```python
from build123d import *

# Parameters (mm, degrees)
SKETCH2_W           = 25
SKETCH2_H           = 42
BOSS_EXTRUDE1_DEPTH = 36
SKETCH4_W           = 23
SKETCH4_H           = 34
CUT_EXTRUDE2_DEPTH  = 61.704200843
FILLET2_R           = 2
SKETCH5_W           = 2.5
SKETCH5_H           = 10
CUT_EXTRUDE3_DEPTH  = 36
FILLET3_R           = 1
FILLET4_R           = 2
SKETCH7_W           = 6.678436395
SKETCH7_H           = 24
BOSS_EXTRUDE2_DEPTH = 2
FILLET5_R           = 2
SKETCH8_W           = 6.678436395
SKETCH8_H           = 2
BOSS_EXTRUDE5_DEPTH = 22
FILLET6_R           = 2
FILLET7_R           = 2
FILLET8_R           = 2
FILLET9_R           = 1
SKETCH10_R          = 2
SKETCH10_R_2        = 4
SKETCH10_R_3        = 1.5
CUT_EXTRUDE5_DEPTH  = 22
SKETCH11_R          = 2
CUT_EXTRUDE6_DEPTH  = 22
SKETCH14_R          = 1.480718613
SKETCH14_R_2        = 1.5
CUT_EXTRUDE8_DEPTH  = 1


with BuildPart() as part:
    # Sketch2 → Boss-Extrude1 (new body)
    with BuildSketch(Plane(origin=(0, 0, 0), x_dir=(1, 0, 0), z_dir=(0, 1, 0))):
        with Locations((12.5, 0)):
            Rectangle(SKETCH2_W, SKETCH2_H)
    extrude(amount=BOSS_EXTRUDE1_DEPTH)

    # Sketch4 → Cut-Extrude2 (cut, through all)
    with BuildSketch(Plane.XY.offset(21)):
        with Locations((13.5, 19)):
            Rectangle(SKETCH4_W, SKETCH4_H)
    extrude(amount=-CUT_EXTRUDE2_DEPTH, mode=Mode.SUBTRACT)

    # Fillet2
    fillet2_edges = [part.edges().sort_by_distance(p)[0] for p in [
        (25, 1, 21),
        (25, 1, -21),
    ]]
    fillet(fillet2_edges, radius=FILLET2_R)

    # Sketch5 → Cut-Extrude3 (cut)
    with BuildSketch(Plane(origin=(2, 0, 0), x_dir=(0, 0, -1), z_dir=(1, 0, 0))):
        with Locations((-19.75, 31)):
            Rectangle(SKETCH5_W, SKETCH5_H)
        with Locations((19.75, 31)):
            Rectangle(SKETCH5_W, SKETCH5_H)
    extrude(amount=-CUT_EXTRUDE3_DEPTH, mode=Mode.SUBTRACT)

    # Fillet3
    fillet3_edges = [part.edges().sort_by_distance(p)[0] for p in [
        (1, 26, 18.5),
        (1, 26, -18.5),
    ]]
    fillet(fillet3_edges, radius=FILLET3_R)

    # Fillet4
    fillet4_edges = [part.edges().sort_by_distance(p)[0] for p in [
        (1, 36, 18.5),
        (1, 36, -18.5),
    ]]
    fillet(fillet4_edges, radius=FILLET4_R)

    # Sketch7 → Boss-Extrude2 (add)
    with BuildSketch(Plane(origin=(2, 0, 0), x_dir=(0, 0, -1), z_dir=(1, 0, 0))):
        with Locations((-24.339218198, 19)):
            Rectangle(SKETCH7_W, SKETCH7_H)
        with Locations((24.339218198, 19)):
            Rectangle(SKETCH7_W, SKETCH7_H)
    extrude(amount=-BOSS_EXTRUDE2_DEPTH)

    # Fillet5
    fillet5_edges = [part.edges().sort_by_distance(p)[0] for p in [
        (1, 7, 27.678436395),
        (1, 7, -27.678436395),
    ]]
    fillet(fillet5_edges, radius=FILLET5_R)

    # Sketch8 → Boss-Extrude5 (add)
    with BuildSketch(Plane(origin=(2, 0, 0), x_dir=(0, 0, -1), z_dir=(1, 0, 0))):
        with Locations((-24.339218198, 30)):
            Rectangle(SKETCH8_W, SKETCH8_H)
        with Locations((24.339218198, 30)):
            Rectangle(SKETCH8_W, SKETCH8_H)
    extrude(amount=BOSS_EXTRUDE5_DEPTH)

    # Fillet6
    fillet6_edges = [part.edges().sort_by_distance(p)[0] for p in [
        (24, 30, 27.678436395),
        (24, 30, 21),
        (24, 30, -21),
        (24, 30, -27.678436395),
    ]]
    fillet(fillet6_edges, radius=FILLET6_R)

    # Fillet7
    fillet7_edges = [part.edges().sort_by_distance(p)[0] for p in [
        (0, 31, 24.339218197),
        (0, 31, -24.339218197),
    ]]
    fillet(fillet7_edges, radius=FILLET7_R)

    # Fillet8
    fillet8_edges = [part.edges().sort_by_distance(p)[0] for p in [
        (0, 0, 0),
    ]]
    fillet(fillet8_edges, radius=FILLET8_R)

    # Fillet9
    fillet9_edges = [part.edges().sort_by_distance(p)[0] for p in [
        (1, 26, 21),
        (1, 26, -21),
    ]]
    fillet(fillet9_edges, radius=FILLET9_R)

    # Sketch10 → Cut-Extrude5 (cut)
    with BuildSketch(Plane(origin=(2, 0, 0), x_dir=(0, 0, -1), z_dir=(1, 0, 0))):
        with Locations(Location((-22.678436395, 13, 0), (0, 0, 90))):
            Circle(SKETCH10_R)
        with Locations(Location((-22.678436395, 23, 0), (0, 0, 90))):
            Circle(SKETCH10_R)
        with Locations((22.678436395, 13)):
            Circle(SKETCH10_R)
        with Locations((22.678436395, 23)):
            Circle(SKETCH10_R)
        with Locations(Location((-11, 25, 0), (0, 0, 90))):
            Circle(SKETCH10_R_2)
        with Locations(Location((-11, 31.5, 0), (0, 0, 90))):
            Circle(SKETCH10_R_3)
        with Locations(Location((-11, 18.5, 0), (0, 0, 90))):
            Circle(SKETCH10_R_3)
        with Locations(Location((-17.5, 25, 0), (0, 0, 90))):
            Circle(SKETCH10_R_3)
        with Locations(Location((-4.5, 25, 0), (0, 0, 90))):
            Circle(SKETCH10_R_3)
        with Locations((11, 18.5)):
            Circle(SKETCH10_R_3)
        with Locations((4.5, 25)):
            Circle(SKETCH10_R_3)
        with Locations((17.5, 25)):
            Circle(SKETCH10_R_3)
        with Locations((11, 31.5)):
            Circle(SKETCH10_R_3)
        with Locations((11, 25)):
            Circle(SKETCH10_R_2)
        with Locations(Location((0, 15, 0), (0, 0, 90))):
            Circle(SKETCH10_R_2)
        with Locations(Location((6.5, 15, 0), (0, 0, 90))):
            Circle(SKETCH10_R_3)
        with Locations(Location((0, 8.5, 0), (0, 0, 90))):
            Circle(SKETCH10_R_3)
        with Locations(Location((0, 21.5, 0), (0, 0, 90))):
            Circle(SKETCH10_R_3)
        with Locations((-6.5, 15)):
            Circle(SKETCH10_R_3)
    extrude(amount=-CUT_EXTRUDE5_DEPTH, mode=Mode.SUBTRACT)

    # Sketch11 → Cut-Extrude6 (cut)
    with BuildSketch(Plane(origin=(0, 31, 0), x_dir=(1, 0, 0), z_dir=(0, 1, 0))):
        with Locations(Location((18, -24.339218197, 0), (0, 0, 270))):
            Circle(SKETCH11_R)
        with Locations(Location((8.25, -24.339218197, 0), (0, 0, 270))):
            Circle(SKETCH11_R)
        with Locations(Location((18, 24.339218197, 0), (0, 0, 180))):
            Circle(SKETCH11_R)
        with Locations(Location((8.25, 24.339218197, 0), (0, 0, 180))):
            Circle(SKETCH11_R)
    extrude(amount=-CUT_EXTRUDE6_DEPTH, mode=Mode.SUBTRACT)

    # Sketch14 → Cut-Extrude8 (cut)
    with BuildSketch(Plane.XZ):
        with Locations(Location((13.12, 8.82, 0), (0, 0, 270))):
            Circle(SKETCH14_R)
        with Locations(Location((19.62, 9.215317048, 0), (0, 0, 270))):
            Circle(SKETCH14_R_2)
        with Locations(Location((6.62, 9.215317048, 0), (0, 0, 270))):
            Circle(SKETCH14_R_2)
        with Locations(Location((12.800679274, 15.312151745, 0), (0, 0, 270))):
            Circle(SKETCH14_R_2)
        with Locations(Location((12.917346355, 2.32, 0), (0, 0, 270))):
            Circle(SKETCH14_R_2)
        with Locations(Location((12.917346355, -2.32, 0), (0, 0, 90))):
            Circle(SKETCH14_R_2)
        with Locations(Location((19.62, -9.215317048, 0), (0, 0, 90))):
            Circle(SKETCH14_R_2)
        with Locations(Location((13.12, -8.82, 0), (0, 0, 90))):
            Circle(SKETCH14_R)
        with Locations(Location((6.62, -9.215317048, 0), (0, 0, 90))):
            Circle(SKETCH14_R_2)
        with Locations(Location((12.800679274, -15.312151745, 0), (0, 0, 90))):
            Circle(SKETCH14_R_2)
    extrude(amount=-CUT_EXTRUDE8_DEPTH, mode=Mode.SUBTRACT)


solid = part.part
```
Geometry check sheet. Reference: the model listing, model coordinates, mm. A direction names the side the tool comes from. Round coordinates to 2 decimals unless told otherwise and drop trailing zeros. Loops run counter-clockwise (first coordinate to the right, second up) from the corner with the lowest first, then second, coordinate; pieces in that order, holes last. Notation, with made-up numbers: (11.25, 17) - (31.25, 17) arc R18 cw to (31.25, 43) - close; hole circle Ø2 at (73.25, 71). An arc over 180 degrees is marked (long way). Use a Markdown table: item, result.
Q1. Access from +Z, -Z, +X, -X, +Y, -Y to the whole of each face (thin tool, end or side, straight path). Record for faces 1 (the flat face through (13, 2, 0)), 2 (the cylindrical face through (0.99, 35.43, -17.9)), 3 (the cylindrical face through (7.195, 0.493, -7.83)), 4 (the flat face through (11, 30, 21)), 5 (the flat face through (13, 29, 24)).
Solutions:
| item | result |
|---|---|
| face 1 | +Z, -Z, +X, +Y |
| face 2 | -Z, +X, -X, +Y |
| face 3 | -Y |
| face 4 | +X, -X, +Y |
| face 5 | +Z, -Z, +X, -Y |
Q2. Cross-section at A-A on z = 0. Record the cut outline in (x, y), plus the area to 3 significant figures.
Solutions:
| item | result |
|---|---|
| outline | (0, 2) arc R2 ccw to (2, 0) - (25, 0) - (25, 2) - (2, 2) - (2, 7) - (0, 7) - close; (0, 10) - (2, 10) - (2, 11) - (0, 11) - close; (0, 19) - (2, 19) - (2, 20) - (0, 20) - close; (0, 23) - (2, 23) - (2, 36) - (0, 36) - close |
| area | 89.1 mm2 |
Q3. Material ranges on line 1 (Z direction, x = 0.75, y = 21.5); line 2 (Y direction, x = 13.75, z = -9.5); line 3 (Y direction, x = 11, z = -16), recorded low to high.
Solutions:
| item | result |
|---|---|
| line 1 | z = -27.68 to -24, -21.36 to -12.94, -9.06 to -1.5, 1.5 to 9.06, 12.94 to 21.36, 24 to 27.68 |
| line 2 | y = 1 to 2 |
| line 3 | y = 0 to 2 |
Q4. Draft check along X on faces 6 (the cylindrical face through (13.565, 0.493, 7.408)), 7 (the cylindrical face through (0.99, 35.4, 17.93)), 8 (the cylindrical face through (0.6, 30.43, 24.29)), 9 (the flat face through (7, 1, 9)). Enter one of: released by +X, released by -X, zero draft, split by the parting line, or undercut.
Solutions:
| item | result |
|---|---|
| face 6 | undercut |
| face 7 | zero draft |
| face 8 | released by -X |
| face 9 | undercut |
Q5. Cross-section at B-B on z = -8.82. Record the cut outline in (x, y), plus the area to 3 significant figures.
Solutions:
| item | result |
|---|---|
| outline | (0, 2) arc R2 ccw to (2, 0) - (5.17, 0) - (5.17, 1) - (8.07, 1) - (8.07, 0) - (11.64, 0) - (11.64, 1) - (14.6, 1) - (14.6, 0) - (18.17, 0) - (18.17, 1) - (21.07, 1) - (21.07, 0) - (25, 0) - (25, 2) - (2, 2) - (2, 21.65) - (0, 21.65) - close; (0, 28.35) - (2, 28.35) - (2, 36) - (0, 36) - close |
| area | 95.0 mm2 |
Q6. Go/stop test with flat-tipped pins: P1, Ø6, axis at x = 9, z = 4, coming from the -Y side; P2, Ø5.5, axis at x = 15, z = -24.5, coming from the -Y side; P3, Ø3, axis at y = 20.5, z = -4, coming from the +X side; P4, Ø1.8, axis at y = 15, z = 6.5, coming from the +X side. Record where each tip stops, or that it passes through.
Solutions:
| item | result |
|---|---|
| P1 | stops at y = 0 |
| P2 | stops at y = 29 |
| P3 | stops at x = 2 |
| P4 | passes through |
Q7. Cross-section at C-C on z = -17.5. Record the cut outline in (x, y), plus the area to 3 significant figures.
Solutions:
| item | result |
|---|---|
| outline | (0, 2) arc R2 ccw to (2, 0) - (25, 0) - (25, 2) - (2, 2) - (2, 23.5) - (0, 23.5) - close; (0, 26.5) - (2, 26.5) - (2, 35.73) - (0, 35.73) - close |
| area | 111 mm2 |
